Answer from the drawing. Dimensions are ordinates in mm from the lowest x, y and z of the part. A direction names the side the tool comes from. Coordinates: 2 decimals unless noted, no trailing zeros. Write each loop counter-clockwise with the first axis right and the second up, starting at its lowest first coordinate (ties: lowest second). Pieces come first, ordered by that corner, then holes.
1) Find the intervals of material crossed by line 1 (X direction, y = 39, z = 35); line 2 (Y direction, x = 37.05, z = 30), in increasing order.
2) Each of these flat-tipped pins is pushed along its axis until it touches: pin 1 Ø0.9 at (x, z) = (5.5, 5.5) entering from +Y; pin 2 Ø2 at (y, z) = (20, 30) entering from +X; pin 3 Ø3 at (x, z) = (6.5, 32) entering from -Y. Where does it stop, or does it pass through?
3) Which of the six approach directions +Z, -Z, +X, -X, +Y, -Y give full straight-line access (tool end or side, diameter ignored) to the marked faces 5, 6 and 7?
4) The part is cut by section C-C (x = 20.5). Determine the outline of the cut face in (y, z) (1 decimal).
5) The part is cut by section A-A (z = 20). Determine the outline of the cut face in (x, y).
6) Determine the mould class of the marked faces 1, 2, 3 and 4 for opening direction Y: +Y half, -Y half, draft (parallel to the pull), parting line (faces both ways), or undercut.
7) The part is cut by section D-D (x = 10). Determine the outline of the cut face in (y, z), then the cut area to 3 significant figures.
8) The part is cut by section B-B (y = 24.7). Determine the outline of the cut face in (x, z).
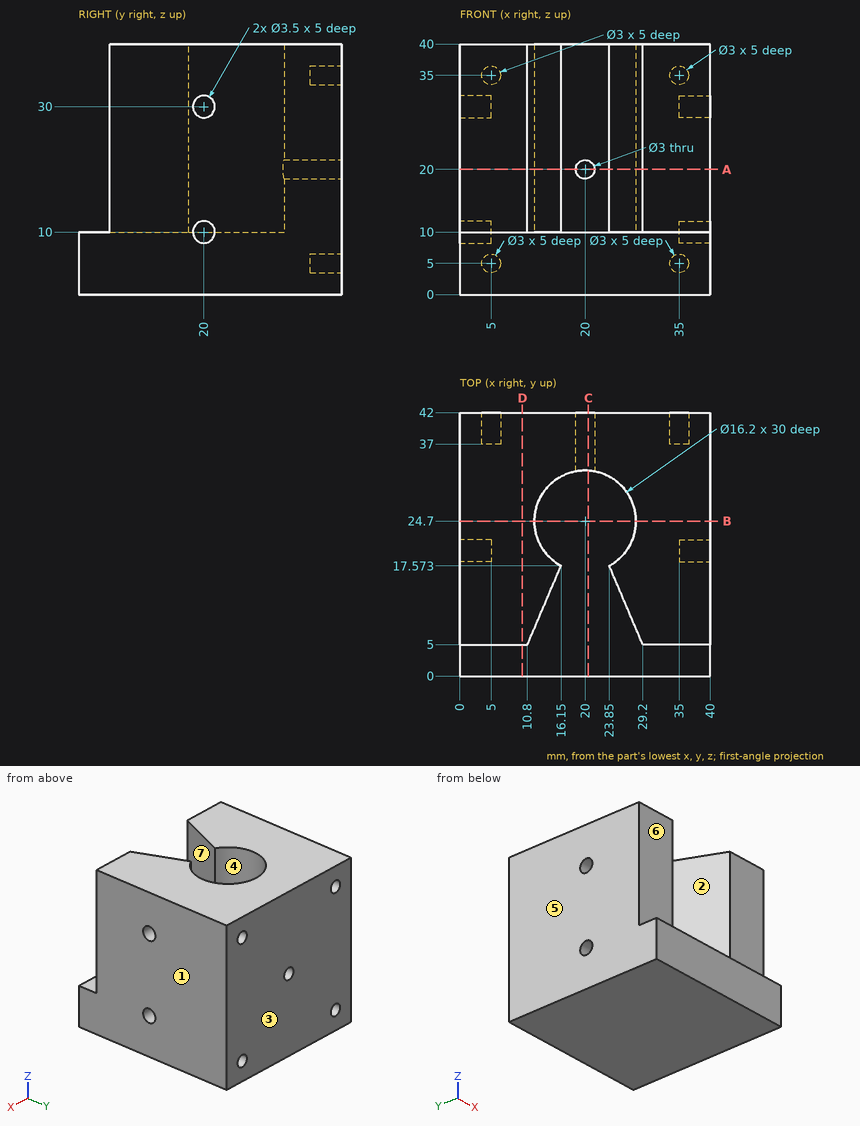
Reported:
1. line 1: x = 0 to 3.5, 6.5 to 33.5, 36.5 to 40
1. line 2: y = 5 to 18.25, 21.75 to 42
2. pin 1: stops at y = 37
2. pin 2: stops at x = 35
2. pin 3: stops at y = 5
3. face 5: +Z, -Z, -X, +Y, -Y
3. face 6: +Z, +X, -X, -Y
3. face 7: +Z, -Y
4. outline: (0, 0) - (42, 0) - (42, 18.6) - (32.8, 18.6) - (32.8, 10) - (0, 10) - close; (32.8, 21.4) - (42, 21.4) - (42, 40) - (32.8, 40) - close
5. outline: (0, 5) - (10.8, 5) - (16.15, 17.57) arc R8.1 cw to (18.5, 32.66) - (18.5, 42) - (0, 42) - close; (21.5, 32.66) arc R8.1 cw to (23.85, 17.57) - (29.2, 5) - (40, 5) - (40, 42) - (21.5, 42) - close
6. face 1: draft
6. face 2: -Y half
6. face 3: +Y half
6. face 4: undercut
7. outline: (0, 0) - (42, 0) - (42, 40) - (5, 40) - (5, 10) - (0, 10) - close
7. area: 1,530 mm2
8. outline: (0, 0) - (40, 0) - (40, 40) - (28.1, 40) - (28.1, 10) - (11.9, 10) - (11.9, 40) - (0, 40) - close
